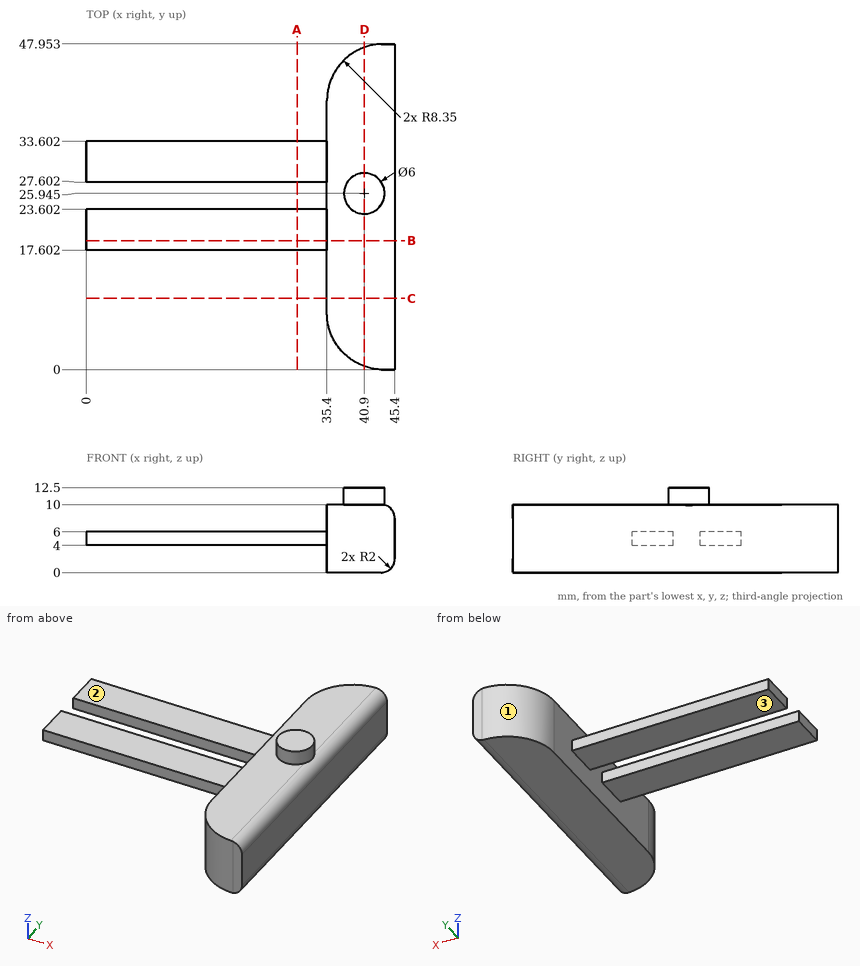
Input: dimensioned drawing with shaded views. Units: mm. Origin: part minimum x, y, z. A direction names the side the tool comes from. Coordinates: 2 decimals unless noted, no trailing zeros. Order: outer loops, then holes, each group sorted by start corner. A loop starts at its lowest first (then second) coordinate and runs counter-clockwise, first axis right, second up.
(1) Section query C-C (y = 10.5). Return the cut outline in (x, z).
(2) Section query A-A (x = 31). Return the cut outline in (y, z).
(3) Material intervals for probe 1 along X at (y, z) = (10, 7.75); probe 2 along Z at (x, y) = (23, 18.5); probe 3 along Z at (x, y) = (42, 35.5), sorted ascending.
(4) Section query D-D (x = 40.9). Return the cut outline in (y, z) (1 decimal).
(5) Access query for the marked faces 1, 2 and 3. Directions: +Z, -Z, +X, -X, +Y, -Y. A direction counts if a zero-diameter tool reaches every point of the face in a straight line with its end or side. Return the directions, or none.
(6) Section query B-B (y = 19). Return the cut outline in (x, z).
(7) First-contact query: pin 1 (2.5 mm diameter, centred on x = 40, y = 12.5, fed in from +Z); pin 2 (4 mm diameter, centred on y = 12, z = 11, fed in from -X); pin 3 (1 mm diameter, centred on x = 24.5, z = 4.5, fed in from -Y). Flat tips, straight axial feed; report the tip coordinate or a pass-through.
Solution:
1. outline: (35.4, 0) - (43.4, 0) arc R2 ccw to (45.4, 2) - (45.4, 8) arc R2 ccw to (43.4, 10) - (35.4, 10) - close
2. outline: (17.6, 4) - (23.6, 4) - (23.6, 6) - (17.6, 6) - close; (27.6, 4) - (33.6, 4) - (33.6, 6) - (27.6, 6) - close
3. probe 1: x = 35.4 to 45.4
3. probe 2: z = 4 to 6
3. probe 3: z = 0 to 10
4. outline: (0.5, 0) - (47.5, 0) - (47.5, 10) - (28.9, 10) - (28.9, 12.5) - (22.9, 12.5) - (22.9, 10) - (0.5, 10) - close
5. face 1: +Z, -Z, -X, +Y
5. face 2: +Z, -X, +Y, -Y
5. face 3: -Z, -X, +Y, -Y
6. outline: (0, 4) - (35.4, 4) - (35.4, 0) - (43.4, 0) arc R2 ccw to (45.4, 2) - (45.4, 8) arc R2 ccw to (43.4, 10) - (35.4, 10) - (35.4, 6) - (0, 6) - close
7. pin 1: stops at z = 10
7. pin 2: stops at x = 35.4
7. pin 3: stops at y = 17.6
